from build123d import *

# Parameters (mm, degrees)
F1_R          = 0.5
F3_DEPTH      = 1
F3_DEPTH_BACK = 1
F5_DEPTH      = 1
F5_DEPTH_BACK = 1
F7_START      = 1
F6_W          = 4
F6_H          = 3.5
F7_DEPTH      = 4


with BuildPart() as f0:
    # F8 (on Front) → F0 (revolve)
    with BuildSketch(Plane.XZ):
        with BuildLine():
            ThreePointArc((5, 100), (3.5355339059, 96.4644660941), (0, 95))
            Line((0, 95), (0, 93))
            Line((0, 93), (4, 93))
            Line((4, 93), (4, 0))
            Line((4, 0), (5, 0))
            Line((5, 0), (5, 100))
        make_face()
    revolve(axis=Axis((0, 0, 94), (0, 0, 1)))

    # F1
    f1_edges = [f0.edges().sort_by_distance(p)[0] for p in [
        (-5, 0, 100),
    ]]
    fillet(f1_edges, radius=F1_R)

    # F2 (on Front) → F3 (join, two sides)
    with BuildSketch(Plane.XZ) as f3_sk:
        Polygon((-50, 0), (50, 0), (4, 50), (4, 95), (-4, 95), (-4, 50), align=None)
    extrude(amount=F3_DEPTH)
    extrude(f3_sk.sketch, amount=-F3_DEPTH_BACK)

    # F4 (on Right) → F5 (join, two sides)
    with BuildSketch(Plane.YZ) as f5_sk:
        Polygon((-50, 0), (50, 0), (4, 50), (4, 85), (-4, 85), (-4, 50), align=None)
    extrude(amount=F5_DEPTH)
    extrude(f5_sk.sketch, amount=-F5_DEPTH_BACK)

    # F6 (on Front) → F7 (cut)
    with BuildSketch(Plane.XZ.offset(F7_START)):
        with Locations((-0.1010205144, 90.0877223398)):
            Rectangle(F6_W, F6_H)
    extrude(amount=F7_DEPTH, mode=Mode.SUBTRACT)


solid = f0.part
CAD build for the part. Positions are in the model's coordinates, mm. A direction names the side the tool comes from. Coordinates: 2 decimals unless noted, no trailing zeros. Loops run counter-clockwise (first coordinate to the right, second up) from the corner with the lowest first, then second, coordinate; pieces in that order, holes last. Notation, with made-up numbers: (55.5, -31) - (110.5, -31) arc R30 ccw to (110.5, -1) - close; hole circle Ø5 at (-8.75, -15.75). An arc over 180 degrees is marked (long way). Use one line per item in the form item = value. Start each with the question number.
1) Tool access for faces 1 (the face through (-1, 2, 43)), 2 (the face through (17, 1, 14)), 3 (the face through (17, -1, 14)), 4 (the face through (-1, -18, 14)): list every direction of +Z, -Z, +X, -X, +Y, -Y with a clear straight run to the whole face (end or side of a thin tool).
2) Band-saw the part on C-C (x = -10.5). Give the cut face in (y, z).
3) Flat gauge pins, fed straight in: pin 1 (0.8 mm diameter, centred on x = -1, y = -4, fed in from +Z); pin 2 (2 mm diameter, centred on x = -14, z = 21.5, fed in from +Y); pin 3 (6 mm diameter, centred on x = 1.5, z = 53, fed in from -Y); pin 4 (22.5 mm diameter, centred on x = -38.5, z = 21, fed in from -Y). Where does each tip first touch, or does it go through?
4) Band-saw the part on D-D (y = -9). Give the cut face in (x, z), and give its area (3 significant figures).
5) Band-saw the part on A-A (z = 14). Give the cut face in (x, y).
6) Band-saw the part on B-B (z = 37). Give the cut face in (x, y), and give its area (3 significant figures).
7) Drill centre lines: L1, parallel to Y at x = -1.5, z = 10; L2, parallel to Y at x = -2, z = 20; L3, parallel to X at y = 6, z = 25. Where is each one in solid material? Low to high. Write a range as from..to.
8) Two-plate mould, pull along Z, no slides. Class faces 5 (the face through (0, 0, 0)), 6 (the face through (1, 17, 14)), 7 (the face through (0, -2, 93)): +Z half, -Z half, draft (parallel to the pull), parting line (faces both ways), or undercut.
Check values:
q1.face_1 = -Z
q1.face_2 = +Z, -Z, +X, +Y
q1.face_3 = +Z, -Z, +X, -Y
q1.face_4 = +Z, -Z, -X, -Y
q2.outline = (-1, 0) - (1, 0) - (1, 42.93) - (-1, 42.93) - close
q3.pin_1 = 97.34
q3.pin_2 = 1
q3.pin_3 = -5
q3.pin_4 = -1
q4.outline = (-1, 0) - (1, 0) - (1, 44.57) - (-1, 44.57) - close
q4.area = 89.1 mm2
q5.outline = (-37.12, -1) - (-4.9, -1) arc R5 ccw to (-1, -4.9) - (-1, -37.12) - (1, -37.12) - (1, -4.9) arc R5 ccw to (4.9, -1) - (37.12, -1) - (37.12, 1) - (4.9, 1) arc R5 ccw to (1, 4.9) - (1, 37.12) - (-1, 37.12) - (-1, 4.9) arc R5 ccw to (-4.9, 1) - (-37.12, 1) - close; hole (-3.87, -1) arc R4 ccw to (-1, -3.87) - (-1, -1) - close; hole (-3.87, 1) - (-1, 1) - (-1, 3.87) arc R4 ccw to start; hole (1, -3.87) arc R4 ccw to (3.87, -1) - (1, -1) - close; hole (1, 1) - (3.87, 1) arc R4 ccw to (1, 3.87) - close
q6.outline = (-15.96, -1) - (-4.9, -1) arc R5 ccw to (-1, -4.9) - (-1, -15.96) - (1, -15.96) - (1, -4.9) arc R5 ccw to (4.9, -1) - (15.96, -1) - (15.96, 1) - (4.9, 1) arc R5 ccw to (1, 4.9) - (1, 15.96) - (-1, 15.96) - (-1, 4.9) arc R5 ccw to (-4.9, 1) - (-15.96, 1) - close; hole (-3.87, -1) arc R4 ccw to (-1, -3.87) - (-1, -1) - close; hole (-3.87, 1) - (-1, 1) - (-1, 3.87) arc R4 ccw to start; hole (1, -3.87) arc R4 ccw to (3.87, -1) - (1, -1) - close; hole (1, 1) - (3.87, 1) arc R4 ccw to (1, 3.87) - close
q6.area = 144 mm2
q7.L1 = -4.77..-3.71, -1..1, 3.71..4.77
q7.L2 = -4.58..-3.46, -1..1, 3.46..4.58
q7.L3 = -1..1
q8.face_5 = -Z half
q8.face_6 = draft
q8.face_7 = undercut
